```python
from build123d import *

# Parameters (mm, degrees)
F1_DEPTH = 50.8
F2_SIZE  = 6.35
F4_D     = 7.9375
F6_D     = 9.525
F6_DEPTH = 19.05
F6_TIP   = 2.8615986981


# Not quite as in the source:
# - a length typed as a fraction of an inch, garbled in the dataset ("3 / 203.2 mm" for 3/8 in), is restored


with BuildPart() as f1:
    # F0 (on Front) → F1 (new body, symmetric)
    with BuildSketch(Plane.XZ):
        Polygon((-106.0025989716, 12.7), (-106.0025989716, -12.7), (97.1974010284, -12.7), (97.1974010284, 6.35), (14.6474010284, 6.35), (14.6474010284, 0), (-93.3025989716, 0), (-93.3025989716, 12.7), align=None)
    extrude(amount=F1_DEPTH, both=True)

    # F2
    f2_edges = [f1.edges().sort_by_distance(p)[0] for p in [
        (97.197401, 0, -12.7),
    ]]
    chamfer(f2_edges, length=F2_SIZE)

    # F4 (through all)
    with Locations(Plane.XY.offset(6.35)):
        with Locations((71.7974010284, 31.75), (71.7974010284, -31.75)):
            Hole(F4_D / 2)

    # F6
    with Locations(Plane(origin=(-106.0025989716, 0, 0), x_dir=(0, -1, 0), z_dir=(-1, 0, 0))):
        with Locations((0, 6.35)):
            Hole(F6_D / 2, depth=F6_DEPTH)
            with Locations((0, 0, -(F6_DEPTH + F6_TIP / 2))):  # 118° drill point
                Cone(0, F6_D / 2, F6_TIP, mode=Mode.SUBTRACT)


solid = f1.part
```
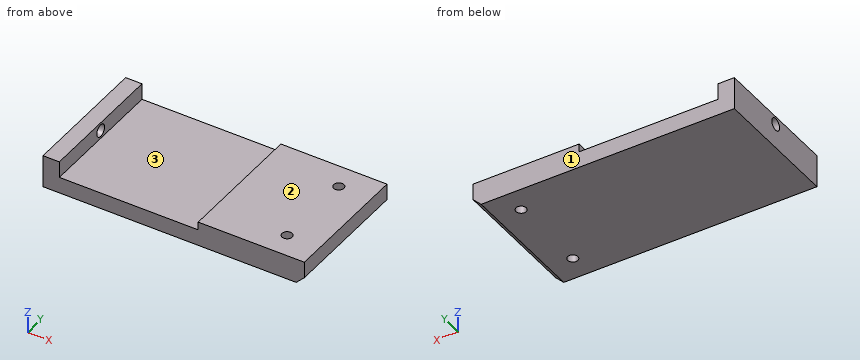
CAD build for the part. Positions are in the model's coordinates, mm. Face numbers are marked on the shaded views. A direction names the side the tool comes from. Give positions to 0.01 mm unless a question says otherwise; leave off trailing zeros. Loops run counter-clockwise (first coordinate to the right, second up) from the corner with the lowest first, then second, coordinate; pieces in that order, holes last. Notation, with made-up numbers: (-12.5, 35.25) - (17.5, 35.25) arc R15 ccw to (17.5, 61.25) - close; hole circle Ø2 at (-8.5, -3.75). An arc over 180 degrees is marked (long way). Put each result on its own line as item: value.
Q1. Slice it at B-B (z = 4.5). Give the cut face in (x, y).
Filled in:
outline: (-106, -50.8) - (-93.3, -50.8) - (-93.3, -4.39) - (-106, -4.39) - close; (-106, 4.39) - (-93.3, 4.39) - (-93.3, 50.8) - (-106, 50.8) - close; (14.65, -50.8) - (97.2, -50.8) - (97.2, 50.8) - (14.65, 50.8) - close; hole circle Ø7.94 at (71.8, -31.75); hole circle Ø7.94 at (71.8, 31.75)
Q2. Tool access for the marked faces 1, 2 and 3: list every direction of +Z, -Z, +X, -X, +Y, -Y with a clear straight run to the whole face (end or side of a thin tool).
Filled in:
face 1: +Z, -Z, +X, -X, +Y
face 2: +Z, +X, +Y, -Y
face 3: +Z, +Y, -Y
Q3. Slice it at A-A (y = -31.75). Give the cut face in (x, z), plus the area to 3 significant figures.
Filled in:
outline: (-106, -12.7) - (67.83, -12.7) - (67.83, 6.35) - (14.65, 6.35) - (14.65, 0) - (-93.3, 0) - (-93.3, 12.7) - (-106, 12.7) - close; (75.77, -12.7) - (90.85, -12.7) - (97.2, -6.35) - (97.2, 6.35) - (75.77, 6.35) - close
area: 3,090 mm²
Q4. Slice it at D-D (x = 27). Give the cut face in (y, z), plus the area to 3 significant figures.
Filled in:
outline: (-50.8, -12.7) - (50.8, -12.7) - (50.8, 6.35) - (-50.8, 6.35) - close
area: 1,940 mm²
Q5. Flat gauge pins, fed straight in: pin 1 (25 mm diameter, centred on x = 51, y = 3, fed in from +Z); pin 2 (1 mm diameter, centred on y = -21.5, z = 7, fed in from +X). Where does each tip first touch, or does it go through?
Filled in:
pin 1: stops at z = 6.35
pin 2: stops at x = -93.3
Q6. Slice it at C-C (y = 0). Give the cut face in (x, z), plus the area to 4 significant figures.
Filled in:
outline: (-106, -12.7) - (90.85, -12.7) - (97.2, -6.35) - (97.2, 6.35) - (14.65, 6.35) - (14.65, 0) - (-93.3, 0) - (-93.3, 1.59) - (-106, 1.59) - close; (-106, 11.11) - (-93.3, 11.11) - (-93.3, 12.7) - (-106, 12.7) - close
area: 3,125 mm²
Q7. Probe line 1 along X through (y, z) = (-33, 0.75); line 2 along Z through (x, y) = (-7, 3.5); line 3 along X through (y, z) = (-5.5, 2.5). List the from-to ranges inside material, lowest first.
Filled in:
line 1: x = -106 to -93.3, 14.65 to 68.03, 75.56 to 97.2
line 2: z = -12.7 to 0
line 3: x = -106 to -93.3, 14.65 to 97.2
